```python
from build123d import *

# Parameters (mm, degrees)
BOSS_EXTRUDE1_DEPTH = 25
RIB1_START          = -28
RIB1_OUTLINE_W      = 55
RIB1_OUTLINE_H      = 8
RIB1_DEPTH          = 28
CUT_EXTRUDE1_DEPTH  = 100
SKETCH2_5_R         = 7.5
CUT_EXTRUDE2_DEPTH  = 20
CHAMFER2_SIZE       = 25


# Read off the part's stored shape, not the designer's step: Rib1
with BuildPart() as part:
    # Sketch1 → Boss-Extrude1 (new, symmetric)
    with BuildSketch(Plane.XY):
        Polygon((27.5, 0), (0, 0), (0, -12), (27.5, -12), (27.5, -40), (95, -40), (95, -28), (45.5, -28), (45.5, 58), (27.5, 58), align=None)
        Polygon((0, -12), (0, 0), (-27.5, 0), (-27.5, 58), (-45.5, 58), (-45.5, -28), (-95, -28), (-95, -40), (-27.5, -40), (-27.5, -12), align=None)
    extrude(amount=BOSS_EXTRUDE1_DEPTH, both=True)

    # Rib1 outline → Rib1 (add)
    with BuildSketch(Plane.XZ.offset(40).offset(RIB1_START)):
        with Locations((0, -7)):
            Rectangle(RIB1_OUTLINE_W, RIB1_OUTLINE_H)
    extrude(amount=RIB1_DEPTH)

    # Sketch4 → Cut-Extrude1 (cut)
    with BuildSketch(Plane.ZY.offset(45.5)):
        with BuildLine():
            ThreePointArc((8, 18), (5.656854249, 23.656854249), (0, 26))
            Line((0, 26), (0, 10))
            ThreePointArc((0, 10), (5.656854249, 12.343145751), (8, 18))
        make_face()
        with BuildLine():
            Line((0, 10), (0, 26))
            ThreePointArc((0, 26), (-8, 18), (0, 10))
        make_face()
        with BuildLine():
            Line((25, 49.224989992), (25, 58))
            Line((25, 58), (-1.3e-08, 58))
            ThreePointArc((-1.3e-08, 58), (13.247648848, 55.742546284), (25, 49.224989992))
        make_face()
        with BuildLine():
            ThreePointArc((-25, 49.224989992), (-13.24764886, 55.74254628), (-1.3e-08, 58))
            Line((-1.3e-08, 58), (-25, 58))
            Line((-25, 58), (-25, 49.224989992))
        make_face()
    extrude(amount=-CUT_EXTRUDE1_DEPTH, mode=Mode.SUBTRACT)

    # Sketch2<5> → Cut-Extrude2 (cut)
    with BuildSketch(Plane.XZ.offset(40)):
        with Locations(Location((-77.5, -7, 0), (0, 0, 270))):
            Circle(SKETCH2_5_R)
        with Locations(Location((77.5, -7, 0), (0, 0, 270))):
            Circle(SKETCH2_5_R)
    extrude(amount=-CUT_EXTRUDE2_DEPTH, mode=Mode.SUBTRACT)

    # Chamfer2
    chamfer2_edges = [part.edges().sort_by_distance(p)[0] for p in [
        (-95, -34, 25),
        (95, -34, 25),
    ]]
    chamfer(chamfer2_edges, length=CHAMFER2_SIZE)


solid = part.part
```
Work out the finished part from the listing and answer in its coordinate system (mm). A direction names the side the tool comes from. Give positions to 0.01 mm unless a question says otherwise; leave off trailing zeros. Write each loop counter-clockwise with the first axis right and the second up, starting at its lowest first coordinate (ties: lowest second). Pieces come first, ordered by that corner, then holes. Notation, with made-up numbers: (2, -3.75) -> (12, -3.75) arc R21 cw to (12, 24.25) -> close; hole circle Ø11 at (6, -40). An arc over 180 degrees is marked (long way). Write item = value, one per line.
Q1. Consider line 1 along X through (y, z) = (-37, -7); line 2 along X through (y, z) = (-19.5, 9.5); line 3 along Y through (x, z) = (-49, -0.5). Determine where each line is inside the solid, lowest interval first.
Computed values:
line_1 = -95 to -85, -70 to 70, 85 to 95
line_2 = -45.5 to -27.5, 27.5 to 45.5
line_3 = -40 to -28
Q2. Section D-D on x = 12.5 is taken. Determine the outline of the cut face in (y, z).
Computed values:
outline = (-40, -11) -> (-12, -11) -> (-12, -25) -> (0, -25) -> (0, 25) -> (-12, 25) -> (-12, -3) -> (-40, -3) -> close
Q3. For a pull along X with two mould halves and no side action, classify faces 1 (the flat face through (65, -28, 0)), 2 (the flat face through (95, -34, -12)), 3 (the flat face through (-27.5, 29, 0)) as pulls with the +X half, pulls with the -X half, needs draft (parallel to the pull), parting line crosses it, or undercut.
Computed values:
face_1 = needs draft
face_2 = pulls with the +X half
face_3 = undercut
Q4. Flat-ended cylindrical pins translate along their axes: pin 1 Ø12 at (x, z) = (7.5, -7.5) entering from +Y; pin 2 Ø8.5 at (x, y) = (13.5, -24) entering from -Z; pin 3 Ø14 at (x, y) = (1, -28) entering from +Z. Find the tip coordinate at first contact, or state that the pin passes through.
Computed values:
pin_1 = 0
pin_2 = -11
pin_3 = -3
Q5. Section B-B on x = -77.5 is taken. Determine the outline of the cut face in (y, z), and give its area (3 significant figures).
Computed values:
outline = (-40, -25) -> (-28, -25) -> (-28, -14.5) -> (-40, -14.5) -> close; (-40, 0.5) -> (-28, 0.5) -> (-28, 17.5) -> (-40, 17.5) -> close
area = 330 mm^2
Q6. Section A-A on y = 4 is taken. Determine the outline of the cut face in (x, z), and give its area (3 significant figures).
Computed values:
outline = (-45.5, -25) -> (-27.5, -25) -> (-27.5, 25) -> (-45.5, 25) -> close; (27.5, -25) -> (45.5, -25) -> (45.5, 25) -> (27.5, 25) -> close
area = 1,800 mm^2
Q7. A tool of negligible diameter and unlimited length cuts with its end or side. For faces 4 (the flat face through (0, -26, -3)), 5 (the flat face through (0, 0, 0)), 6 (the flat face through (-45.5, 6, 0)), 7 (the flat face through (0, -26, -11)), from which of +Z, -Z, +X, -X, +Y, -Y can it reach the whole face along a straight path? Write none if from no direction.
Computed values:
face_4 = +Z, -Y
face_5 = +Z, -Z, +Y
face_6 = +Z, -Z, -X, +Y
face_7 = -Z, -Y
Q8. Section C-C on x = 42.5 is taken. Determine the outline of the cut face in (y, z).
Computed values:
outline = (-40, -25) -> (49.22, -25) arc R40 ccw to (49.22, 25) -> (-40, 25) -> close; hole circle Ø16 at (18, 0)
